```python
from build123d import *

# Parameters (mm, degrees)
SKETCH1_W           = 100
SKETCH1_H           = 120
BOSS_EXTRUDE1_DEPTH = 3
SKETCH2_W           = 75.6
SKETCH2_H           = 113.6
BOSS_EXTRUDE2_DEPTH = 3
SKETCH3_R           = 1.6
CUT_EXTRUDE1_DEPTH  = 79.160092119


with BuildPart() as part:
    # Sketch1 → Boss-Extrude1 (new body)
    with BuildSketch(Plane(origin=(0, 0, 0), x_dir=(1, 0, 0), z_dir=(0, 1, 0))):
        Rectangle(SKETCH1_W, SKETCH1_H)
    extrude(amount=BOSS_EXTRUDE1_DEPTH)

    # Sketch2 → Boss-Extrude2 (add)
    with BuildSketch(Plane(origin=(0, 3, 0), x_dir=(1, 0, 0), z_dir=(0, 1, 0))):
        with Locations((-5.8, 0)):
            Rectangle(SKETCH2_W, SKETCH2_H)
    extrude(amount=BOSS_EXTRUDE2_DEPTH)

    # Sketch3 → Cut-Extrude1 (cut, through all)
    with BuildSketch(Plane(origin=(0, 3, 0), x_dir=(1, 0, 0), z_dir=(0, 1, 0))):
        with Locations(Location((41, -50, 0), (0, 0, 270))):
            Circle(SKETCH3_R)
        with Locations(Location((41, 50, 0), (0, 0, 270))):
            Circle(SKETCH3_R)
        with Locations(Location((-47, -50, 0), (0, 0, 270))):
            Circle(SKETCH3_R)
        with Locations(Location((-47, 50, 0), (0, 0, 270))):
            Circle(SKETCH3_R)
    extrude(amount=-CUT_EXTRUDE1_DEPTH, mode=Mode.SUBTRACT)


solid = part.part
```
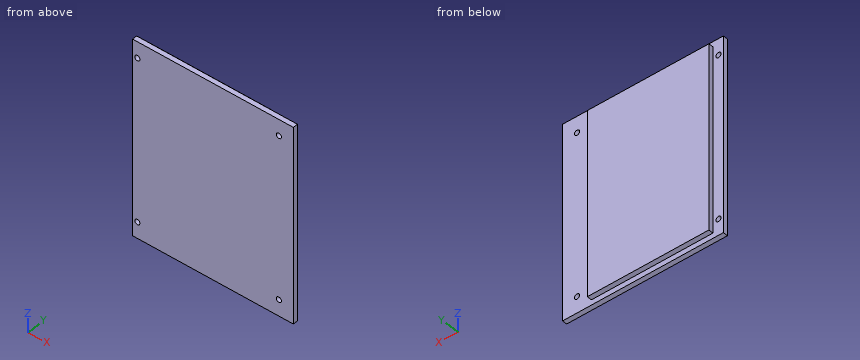
Work out the finished part from the listing and answer in its coordinate system (mm). Give positions to 0.01 mm unless a question says otherwise; leave off trailing zeros. Loops run counter-clockwise (first coordinate to the right, second up) from the corner with the lowest first, then second, coordinate; pieces in that order, holes last. Notation, with made-up numbers: (60.25, 73.25) -> (115.25, 73.25) arc R17 ccw to (115.25, 99.25) -> close; hole circle Ø9 at (-12, 41). An arc over 180 degrees is marked (long way). Put each result on its own line as item: value. Start each with the question number.
Item 1: The part is cut by section B-B (z = -50). Give the vertices of the cut face in (x, y).
Item 2: The part is cut by section D-D (y = 4). Give the vertices of the cut face in (x, z), then the cut area to 3 significant figures.
Item 3: The part is cut by section C-C (z = -5). Give the vertices of the cut face in (x, y), then the cut area to 3 significant figures.
Item 4: Find the intervals of material crossed by L1, parallel to X at y = 1.7, z = 50; L2, parallel to X at y = 3.5, z = -14; L3, parallel to Z at x = -41.5, y = 5.05, in increasing order. Write a range as [from, to].
Item 5: Each of these flat-tipped pins is pushed along its axis until it touches: P1, Ø0.9, axis at y = 4, z = -22, coming from the +X side; P2, Ø0.9, axis at x = 8.5, y = 4, coming from the -Z side; P3, Ø1.5, axis at y = 4, z = 18.5, coming from the -X side. Where does it stop, or does it pass through?
Item 6: The part is cut by section A-A (x = -47). Give the vertices of the cut face in (y, z).
Answers below:
1. outline: (-50, 0) -> (-48.6, 0) -> (-48.6, 3) -> (-50, 3) -> close; (-45.4, 0) -> (39.4, 0) -> (39.4, 3) -> (32, 3) -> (32, 6) -> (-43.6, 6) -> (-43.6, 3) -> (-45.4, 3) -> close; (42.6, 0) -> (50, 0) -> (50, 3) -> (42.6, 3) -> close
2. outline: (-43.6, -56.8) -> (32, -56.8) -> (32, 56.8) -> (-43.6, 56.8) -> close
2. area: 8,590 mm2
3. outline: (-50, 0) -> (50, 0) -> (50, 3) -> (32, 3) -> (32, 6) -> (-43.6, 6) -> (-43.6, 3) -> (-50, 3) -> close
3. area: 527 mm2
4. L1: [-50, -48.6], [-45.4, 39.4], [42.6, 50]
4. L2: [-43.6, 32]
4. L3: [-56.8, 56.8]
5. P1: x = 32
5. P2: z = -56.8
5. P3: x = -43.6
6. outline: (0, -60) -> (3, -60) -> (3, -51.6) -> (0, -51.6) -> close; (0, -48.4) -> (3, -48.4) -> (3, 48.4) -> (0, 48.4) -> close; (0, 51.6) -> (3, 51.6) -> (3, 60) -> (0, 60) -> close
